Work out the finished part from the listing and answer in its coordinate system (mm). A direction names the side the tool comes from. Round coordinates to 2 decimals unless told otherwise and drop trailing zeros. Order: outer loops, then holes, each group sorted by start corner. A loop starts at its lowest first (then second) coordinate and runs counter-clockwise, first axis right, second up.
Autodesk Inventor part; units mm, degrees
ref_plane "Work Plane1" through (-56.3599, 0, 22) normal (0, 0, -1) x (-1, 0, 0)
ref_plane "YZ Plane" through (0, 0, 0) normal (1, 0, 0) x (0, 1, 0)
ref_plane "XZ Plane" through (0, 0, 0) normal (0, 1, 0) x (-1, 0, 0)
ref_plane "Work Plane1" through (-56.3599, 0, 22) normal (0, 0, -1) x (-1, 0, 0)
sketch "Sketch1" plane through (-56.3599, 0, 22) normal (0, 0, -1) x (-1, 0, 0)
  line L0 (-4.0299, -0.3538) -> (-2.2322, 1.4439) construction
  arc A0 (-1.4439, 2.2322) -> (-2.2322, 1.4439) centre (-0.9299, 0.9299) ccw construction
  line L1 (-1.4439, 2.2322) -> (0.3538, 4.0299) construction
  line L2 (-37.8299, 42.8299) -> (-37.8299, 37.8299) construction
  line L3 (-37.8299, 37.8299) -> (-42.9208, 37.8299) construction
  line L4 (-37.8299, 42.2137) -> (-37.8299, 45.8299) construction
  line L5 (-37.8299, 45.8299) -> (-4.0299, 45.8299) construction
  line L6 (-4.0299, 45.8299) -> (-4.0299, 42.2137) construction
  line L7 (-4.0299, 4.0299) -> (0.3538, 4.0299)
  circle A1 centre (-20.9299, 20.9299) radius 17.5
  line L8 (-20.9299, 58.9723) -> (17.1124, 20.9299) construction
  line L9 (17.1124, 20.9299) -> (-20.9299, -17.1124) construction
  line L10 (-20.9299, -17.1124) -> (-58.9723, 20.9299) construction
  line L11 (-58.9723, 20.9299) -> (-20.9299, 58.9723) construction
  line L12 (-20.9299, 58.9723) -> (-20.9299, -17.1124) construction
  line L13 (17.1124, 20.9299) -> (-58.9723, 20.9299) construction
  line L14 (-20.9299, 58.9723) -> (32.8701, 58.9723) construction
  line L15 (-43.4299, 43.4299) -> (1.5701, 43.4299) construction
  line L16 (1.5701, 43.4299) -> (1.5701, -1.5701) construction
  line L17 (1.5701, -1.5701) -> (-43.4299, -1.5701) construction
  line L18 (-43.4299, -1.5701) -> (-43.4299, 43.4299) construction
  line L19 (-43.4299, 43.4299) -> (1.5701, -1.5701) construction
  line L20 (1.5701, 43.4299) -> (-43.4299, -1.5701) construction
  line L21 (-43.4299, 5.3876) -> (-43.4299, 36.4723)
  line L22 (-43.4299, 36.4723) -> (-36.4723, 43.4299)
  line L23 (-36.4723, 43.4299) -> (-5.3876, 43.4299)
  line L24 (-5.3876, 43.4299) -> (1.5701, 36.4723)
  line L25 (1.5701, 36.4723) -> (1.5701, 5.3876)
  line L26 (1.5701, 5.3876) -> (-5.3876, -1.5701)
  line L27 (-5.3876, -1.5701) -> (-36.4723, -1.5701)
  line L28 (-36.4723, -1.5701) -> (-43.4299, 5.3876)
  line L29 (-4.0299, 42.2137) -> (-37.8299, 42.2137)
  line L30 (-4.0299, -0.3538) -> (-4.0299, 4.0299)
  circle A2 centre (-20.9299, 20.9299) radius 1.5
  line L31 (-10.9299, 10.9299) -> (-30.9299, 10.9299) construction
  line L32 (-30.9299, 10.9299) -> (-30.9299, 30.9299) construction
  line L33 (-30.9299, 30.9299) -> (-10.9299, 30.9299) construction
  line L34 (-10.9299, 30.9299) -> (-10.9299, 10.9299) construction
  line L35 (-10.9299, 10.9299) -> (-30.9299, 30.9299) construction
  line L36 (-30.9299, 10.9299) -> (-10.9299, 30.9299) construction
  circle A3 centre (-30.9299, 30.9299) radius 1.4
  circle A4 centre (-30.9299, 10.9299) radius 1.4
  circle A5 centre (-10.9299, 10.9299) radius 1.4
  line L37 (-45.8299, 37.8299) -> (-42.0723, 37.8299) construction
  line L38 (-42.1723, 37.7299) -> (-45.8299, 37.7299)
  line L39 (-45.8299, 37.7299) -> (-45.8299, 4.1299)
  line L40 (-45.8299, 4.1299) -> (-42.1723, 4.1299)
  line L41 (-42.1723, 4.1299) -> (-42.1723, 37.7299)
  line L42 (-45.8299, 4.0299) -> (-42.0723, 4.0299) construction
  line L43 (-45.8299, 37.8299) -> (-42.0723, 37.8299)
  line L44 (-37.7299, 45.8299) -> (-4.1299, 45.8299)
  line L45 (-4.1299, 45.8299) -> (-4.1299, 42.1723)
  line L46 (-4.1299, 42.1723) -> (-37.7299, 42.1723)
  line L47 (-37.7299, 42.1723) -> (-37.7299, 45.8299)
  line L48 (0.4701, 37.8299) -> (0.4701, 4.0299) construction
  line L49 (0.4701, 4.0299) -> (3.9701, 4.0299) construction
  line L50 (3.9701, 37.8299) -> (3.9701, 4.0299) construction
  line L51 (0.4701, 37.8299) -> (3.9701, 37.8299) construction
  line L52 (-45.8299, -3.9701) -> (-4.0299, -3.9701) construction
  line L53 (0.3124, 37.7299) -> (3.9701, 37.7299)
  line L54 (3.9701, 37.7299) -> (3.9701, 4.1299)
  line L55 (3.9701, 4.1299) -> (0.3124, 4.1299)
  line L56 (0.3124, 4.1299) -> (0.3124, 37.7299)
  line L57 (-4.1713, -0.3538) -> (-37.7299, -0.3538)
  line L58 (-37.7299, -0.3538) -> (-37.7299, -3.9701)
  line L59 (-37.7299, -3.9701) -> (-4.1713, -3.9701)
  line L60 (-4.1713, -3.9701) -> (-4.1713, -0.3538)
  point P0 (-37.8299, 4.0299)
  dimension "d18" = 53.8
  dimension "d19" = 45
  dimension "d20" = 53.8
  dimension "d21" = 45
  dimension "d22" = 45
  dimension "d30" = 20
  dimension "d31" = 20
  dimension "d32" = 2.8
  dimension "d33" = 2.8
  dimension "d34" = 2.8
  dimension "d35" = 3
  dimension "d36" = 0.1
  dimension "d37" = 0.1
  dimension "d38" = 0.1
  dimension "d39" = 0.1
extrude "Extrusion1" add sketch "Sketch1" along normal blind 10 contours L30 L26 L57 L28 L41 L22 L46 L24 L56 L7 | L7 L26 L30 | L56 L24 L25 L26 | L26 L25 L24 L53 L54 L55 | L60 L59 L58 L57 L28 L27 L26 | L26 L27 L28 L57 | L46 L22 L29 L24 | L24 L29 L45 | L40 L39 L38 L22 L21 L28 | L28 L21 L22 L41 | L29 L22 L23 L24 | L24 L23 L22 L29 L47 L44 L45 | L47 L29 L22 | A1 | A2 | A3 | A4 | A5
sketch "Skizze4" plane through (-56.3599, 0, 12) normal (0, 0, -1) x (-1, 0, 0)
  line L0 (-37.7299, 42.1723) -> (-42.1723, 37.7299)
  line L1 (-42.1723, 37.7299) -> (-45.8299, 37.7299)
  line L2 (-45.8299, 37.7299) -> (-45.8299, 4.1299) construction
  line L3 (-45.8299, 4.1299) -> (-42.1723, 4.1299)
  line L4 (-42.1723, 4.1299) -> (-37.6885, -0.3538)
  line L5 (-37.6885, -0.3538) -> (-37.7299, -0.3538)
  line L6 (-37.7299, -0.3538) -> (-37.7299, -3.9701)
  line L7 (-37.7299, -3.9701) -> (-4.1713, -3.9701) construction
  line L8 (-4.1713, -3.9701) -> (-4.1713, -0.3538)
  line L9 (-4.1713, -0.3538) -> (0.3124, 4.1299)
  line L10 (0.3124, 4.1299) -> (3.9701, 4.1299)
  line L11 (3.9701, 4.1299) -> (3.9701, 37.7299) construction
  line L12 (3.9701, 37.7299) -> (0.3124, 37.7299)
  line L13 (0.3124, 37.7299) -> (-4.1299, 42.1723)
  line L14 (-4.1299, 42.1723) -> (-4.1299, 45.8299)
  line L15 (-4.1299, 45.8299) -> (-37.7299, 45.8299) construction
  line L16 (-37.7299, 45.8299) -> (-37.7299, 42.1723)
  line L17 (-37.9299, 46.0299) -> (-3.9299, 46.0299) construction
  line L18 (-3.9299, 46.0299) -> (-3.9299, 42.2551)
  line L19 (-3.9299, 42.2551) -> (0.3953, 37.9299)
  line L20 (0.3953, 37.9299) -> (4.1701, 37.9299)
  line L21 (4.1701, 37.9299) -> (4.1701, 3.9299) construction
  line L22 (4.1701, 3.9299) -> (0.3953, 3.9299)
  line L23 (0.3953, 3.9299) -> (-3.9713, -0.4367)
  line L24 (-3.9713, -0.4367) -> (-3.9713, -4.1701)
  line L25 (-3.9713, -4.1701) -> (-37.9299, -4.1701) construction
  line L26 (-37.9299, -4.1701) -> (-37.9299, -0.3953)
  line L27 (-37.9299, -0.3953) -> (-42.2551, 3.9299)
  line L28 (-42.2551, 3.9299) -> (-46.0299, 3.9299)
  line L29 (-46.0299, 3.9299) -> (-46.0299, 37.9299) construction
  line L30 (-46.0299, 37.9299) -> (-42.2551, 37.9299)
  line L31 (-42.2551, 37.9299) -> (-37.9299, 42.2551)
  line L32 (-37.9299, 42.2551) -> (-37.9299, 46.0299)
  line L33 (-45.8299, 37.7299) -> (-45.8299, 37.9299)
  line L34 (-4.1299, 45.8299) -> (-37.7299, 45.8299)
  line L35 (-37.7299, 45.8299) -> (-37.9299, 45.8299)
  line L36 (-4.1299, 45.8299) -> (-3.9299, 45.8299)
  line L37 (3.9701, 37.7299) -> (3.9701, 37.9299)
  line L38 (3.9701, 4.1299) -> (3.9701, 37.7299)
  line L39 (3.9701, 4.1299) -> (3.9701, 3.9299)
  line L40 (-4.1713, -3.9701) -> (-3.9713, -3.9701)
  line L41 (-37.7299, -3.9701) -> (-37.9299, -3.9701)
  line L42 (-45.8299, 4.1299) -> (-45.8299, 3.9299)
  point P0 (-56.3599, 0)
  dimension "d40" = 0.2
extrude "IM_offset" add sketch "Skizze4" against normal up to surface (10 mm away)
ref_plane "Arbeitsebene5" through (-35.4299, 3.9299, 22) normal (-1, 0, 0) x (0, 0, 1)
ref_plane "Arbeitsebene6" through (-18.4299, 20.9299, 22) normal (0, 1, 0) x (-1, 0, 0)
sketch "Sketch33" plane through (-56.3599, 0, 12) normal (0, 0, -1) x (-1, 0, 0)
  circle A0 centre (-20.9299, 20.9299) radius 15.24 construction
  circle A1 centre (-20.9299, 20.9299) radius 15.14 construction
  line L0 (-12.0272, 5.7899) -> (-29.8327, 5.7899)
  line L1 (-38.4929, 20.7899) -> (-29.5902, 36.2099)
  line L2 (-12.2697, 36.2099) -> (-3.3669, 20.7899)
  line L3 (-42.2551, 3.9299) -> (-45.8299, 3.9299)
  arc A2 (-12.0272, 5.7899) -> (-3.3669, 20.7899) centre (-12.0272, 15.7899) ccw
  arc A3 (-38.4929, 20.7899) -> (-29.8327, 5.7899) centre (-29.8327, 15.7899) ccw
  arc A4 (-12.2697, 36.2099) -> (-29.5902, 36.2099) centre (-20.9299, 31.2099) ccw
  point P0 (-56.3599, 0)
  point P1 (5.2933, 5.7899)
  point P2 (-47.1532, 5.7899)
  point P3 (-20.9299, 51.2099)
  dimension "d184" = 0.1
  dimension "d185" = 0
  dimension "d186" = 10
extrude "Extrusion27" cut sketch "Sketch33" against normal blind 10
sketch "Sketch34" plane through (-56.3599, 0, 22) normal (0, 0, 1) x (1, 0, 0)
  arc A0 (29.8327, 5.7899) -> (38.4929, 20.7899) centre (29.8327, 15.7899) ccw
  line L0 (29.8327, 5.7899) -> (12.0272, 5.7899)
  arc A1 (3.3669, 20.7899) -> (12.0272, 5.7899) centre (12.0272, 15.7899) ccw
  line L1 (3.3669, 20.7899) -> (12.2697, 36.2099)
  arc A2 (29.5902, 36.2099) -> (12.2697, 36.2099) centre (20.9299, 31.2099) ccw
  line L2 (29.5902, 36.2099) -> (38.4929, 20.7899)
  line L3 (3.9713, -3.9701) -> (37.9299, -3.9701)
  line L4 (37.9299, -3.9701) -> (37.9299, -0.3953)
  line L5 (37.9299, -0.3953) -> (42.2551, 3.9299)
  line L6 (42.2551, 3.9299) -> (45.8299, 3.9299)
  line L7 (45.8299, 3.9299) -> (45.8299, 37.9299)
  line L8 (45.8299, 37.9299) -> (42.2551, 37.9299)
  line L9 (42.2551, 37.9299) -> (37.9299, 42.2551)
  line L10 (37.9299, 42.2551) -> (37.9299, 45.8299)
  line L11 (37.9299, 45.8299) -> (3.9299, 45.8299)
  line L12 (3.9299, 45.8299) -> (3.9299, 42.2551)
  line L13 (3.9299, 42.2551) -> (-0.3953, 37.9299)
  line L14 (-0.3953, 37.9299) -> (-3.9701, 37.9299)
  line L15 (-3.9701, 37.9299) -> (-3.9701, 3.9299)
  line L16 (-3.9701, 3.9299) -> (-0.3953, 3.9299)
  line L17 (-0.3953, 3.9299) -> (3.9713, -0.4367)
  line L18 (3.9713, -0.4367) -> (3.9713, -3.9701)
  circle A3 centre (20.9299, 20.9299) radius 13.5001 construction
  circle A4 centre (20.9299, 20.9299) radius 13.4001
  line L19 (12.0272, 7.5298) -> (29.8327, 7.5298)
  arc A5 (29.8327, 7.5298) -> (36.9861, 19.92) centre (29.8327, 15.7899) ccw
  line L20 (36.9861, 19.92) -> (28.0834, 35.34)
  arc A6 (28.0834, 35.34) -> (13.7765, 35.34) centre (20.9299, 31.2099) ccw
  line L21 (13.7765, 35.34) -> (4.8737, 19.92)
  arc A7 (4.8737, 19.92) -> (12.0272, 7.5298) centre (12.0272, 15.7899) ccw
  point P0 (56.3599, 0)
  dimension "d189" = 0.1
extrude "Extrusion28" add sketch "Sketch34" along normal blind 1.5 contours L0 A1 L1 A2 L2 A0 | L18 L17 L16 L15 L14 L13 L12 L11 L10 L9 L8 L7 L6 L5 L4 L3
sketch "Sketch35" plane through (-52.3885, -3.9701, 12) normal (0, -1, 0) x (1, 0, 0)
  line L0 (0, 0) -> (0, 11.5)
  line L1 (0, 0) -> (33.9586, 0)
  line L2 (33.9586, 0) -> (33.9586, 11.5)
  line L3 (0, 11.5) -> (33.9586, 11.5)
  circle A0 centre (16.9586, 4.104) radius 1.4
  point P0 (52.3885, -12)
  dimension "d192" = 2.8
extrude "Extrusion29" cut sketch "Sketch35" along normal mid plane 30 contours A0
pattern_circular "Circular Pattern2" count 3 over 360 about axis through (-35.4299, 20.9299, 22) along (0, 0, 1) of "Extrusion29"
properties part number "20_Cube_Insert_Filter_25mm"
Item 1: A tool of negligible diameter and unlimited length cuts with its end or side. For faces 5 (the face through (-12, 37.93, 18)), 6 (the face through (-36, 7.53, 23)), 7 (the face through (-18.43, -2, 18)), 8 (the face through (-34.137, 0.842, 15.568)), 9 (the face through (-52.919, 10.663, 16.93)), from which of +Z, -Z, +X, -X, +Y, -Y can it reach the whole face along a straight path? Write none if from no direction.
Item 2: Find section D-D (z = 16.75). State how many separate pieces and enclosed holes the cut face has, plus the area to 3 significant figures.
Item 3: Find the intervals of material crossed by line 1 along X through (y, z) = (43.5, 18.25); line 2 along X through (y, z) = (12.5, 18.5); line 3 along Y through (x, z) = (-12.5, 16.75), in increasing order.
Item 4: Given pin 1 (1.8 mm diameter, centred on y = -2.5, z = 17.5, fed in from -X); pin 2 (1.8 mm diameter, centred on x = -12.5, z = 19.5, fed in from -Y); pin 3 (4 mm diameter, centred on y = -1.5, z = 18.5, fed in from +X); pin 4 (1.5 mm diameter, centred on x = -51, y = 16, fed in from +Z), each flat-ended and moving along its own axis, determine where each tip first touches the part or whether it passes through.
Item 5: Find section C-C (z = 19.5). Write down the section's boundary in (x, y).
Item 6: Find section B-B (y = 17.5). Write down the section's boundary in (x, z), plus the area to 3 significant figures.
Item 7: Find section A-A (x = -45.5). Write down the section's boundary in (y, z), plus the area to 3 significant figures.
Item 8: For a pull along X with two mould halves and no side action, classify faces 1 (the face through (-60.33, 21, 18)), 2 (the face through (-59, 3.93, 18)), 3 (the face through (-16.237, 40.062, 17.67)), 4 (the face through (-54.323, 33.12, 15.252)) as released by +X, released by -X, zero draft, split by the parting line, or undercut.
Model answer:
1. face 5: +Z, -Z, +X, +Y
1. face 6: +Z, -Z
1. face 7: +Z, -Z, +X, -Y
1. face 8: -Y
1. face 9: -Z
2. separate pieces: 3
2. enclosed holes: 0
2. area: 1,190 mm2
3. line 1: x = -52.43 to -18.43
3. line 2: x = -60.33 to -53.78, -17.08 to -10.53
3. line 3: y = 3.93 to 32.73, 35.6 to 37.93
4. pin 1: stops at x = -52.39
4. pin 2: stops at y = 3.93
4. pin 3: stops at x = -17.53
4. pin 4: passes through
5. outline: (-60.33, 3.93) - (-56.76, 3.93) - (-52.39, -0.44) - (-52.39, -3.97) - (-18.43, -3.97) - (-18.43, -0.4) - (-14.1, 3.93) - (-10.53, 3.93) - (-10.53, 37.93) - (-14.1, 37.93) - (-18.43, 42.26) - (-18.43, 45.83) - (-52.43, 45.83) - (-52.43, 42.26) - (-56.76, 37.93) - (-60.33, 37.93) - close; hole (-52.99, 20.79) arc R10 ccw to (-44.33, 5.79) - (-26.53, 5.79) arc R10 ccw to (-17.87, 20.79) - (-26.77, 36.21) arc R10 ccw to (-44.09, 36.21) - close
6. outline: (-60.33, 12) - (-54.19, 12) - (-54.19, 22) - (-52.41, 22) - (-52.41, 23.5) - (-60.33, 23.5) - close; (-18.45, 22) - (-16.67, 22) - (-16.67, 12) - (-10.53, 12) - (-10.53, 23.5) - (-18.45, 23.5) - close
6. area: 147 mm2
7. outline: (-3.97, 12) - (5.86, 12) - (5.86, 22) - (7.61, 22) - (7.61, 23.5) - (-3.97, 23.5) - close; (30.29, 22) - (33.77, 22) - (33.77, 12) - (45.83, 12) - (45.83, 23.5) - (30.29, 23.5) - close
7. area: 260 mm2
8. face 1: released by -X
8. face 2: zero draft
8. face 3: released by +X
8. face 4: undercut
